Could you check a few things on this model? Use its own coordinates, in mm. A direction names the side the tool comes from. Round coordinates to 2 decimals unless told otherwise and drop trailing zeros. Order: outer loops, then holes, each group sorted by start corner. A loop starts at its lowest first (then second) coordinate and runs counter-clockwise, first axis right, second up. Notation, with made-up numbers: M 81,88.5 L 118,88.5 A21 ccw 118,92.5 Z; hole C 63.25,53.5 d4. An arc over 180 degrees is marked long. Write each question's results on one line, items separated by ' | '. Start each with the question number.
1. We'd pull the mould along Y, two halves only. Please class faces 3 (the flat face through (0, -6.35, 25)), 4 (the cylindrical face through (-2.75, -12.4, 25.05)), 5 (the flat face through (-6, 3, 0)): released by +Y, released by -Y, zero draft, split by the parting line, or undercut.
2. For faces 1 (the flat face through (-6, 3, 50.8)), 2 (the flat face through (5.525, -3.131, 25.044)), which set-ups out of +Z, -Z, +X, -X, +Y, -Y let a thin tool reach every point of the face, with its end or its side?
3. Suppose I cut it at A-A on z = 20.5. Write out the boundary of the cut face in (x, y), and give its area (3 significant figures).
4. Suppose I cut it at B-B on x = 0. Write out the boundary of the cut face in (y, z), and give its area (3 significant figures).
5. I'm going to push flat-ended pins straight in: pin 1 (2 mm diameter, centred on y = -1.5, z = 16, fed in from -X); pin 2 (10 mm diameter, centred on x = 8.5, z = 39, fed in from -Y); pin 3 (1 mm diameter, centred on x = 5.5, z = 20.5, fed in from -Y). Where does each tip first touch, or does it pass through?
6. Please list where these lines run through material, in increasing order: L1, parallel to Y at x = -6, z = 8; L2, parallel to Y at x = -11, z = 14.5; L3, parallel to X at y = 1.75, z = 43.5.
from build123d import *

# Parameters (mm, degrees)
F0_R     = 12.7
F1_DEPTH = 50.8
F2_SIZE  = 0.254


with BuildPart() as f1:
    # F0 (on Top) → F1 (new body)
    with BuildSketch(Plane.XY):
        Circle(F0_R)
        Polygon((-3.666174, 6.35), (3.666174, 6.35), (7.332348, 0), (3.666174, -6.35), (-3.666174, -6.35), (-7.332348, 0), align=None, mode=Mode.SUBTRACT)
    extrude(amount=F1_DEPTH)

    # F2
    f2_edges = [f1.edges().sort_by_distance(p)[0] for p in [
        (-12.7, 0, 50.8),
        (-12.7, 0, 0),
    ]]
    chamfer(f2_edges, length=F2_SIZE)


solid = f1.part
Filled sheet:
1) face 3: undercut | face 4: split by the parting line | face 5: zero draft
2) face 1: +Z, +X, -X, +Y, -Y | face 2: +Z, -Z
3) outline: C 0,0 d25.4; hole M -7.33,0 L -3.67,-6.35 L 3.67,-6.35 L 7.33,0 L 3.67,6.35 L -3.67,6.35 Z | area: 367 mm^2
4) outline: M -12.7,0.25 L -12.45,0 L -6.35,0 L -6.35,50.8 L -12.45,50.8 L -12.7,50.55 Z; M 6.35,0 L 12.45,0 L 12.7,0.25 L 12.7,50.55 L 12.45,50.8 L 6.35,50.8 Z | area: 645 mm^2
5) pin 1: stops at x = -12.69 | pin 2: stops at y = -12.21 | pin 3: stops at y = -11.67
6) L1: y = -11.19 to -2.31, 2.31 to 11.19 | L2: y = -6.35 to 6.35 | L3: x = -12.58 to -6.32, 6.32 to 12.58
